Could you check a few things on this model? Use its own coordinates, in mm. A direction names the side the tool comes from. Round coordinates to 2 decimals unless told otherwise and drop trailing zeros. Loops run counter-clockwise (first coordinate to the right, second up) from the corner with the lowest first, then second, coordinate; pieces in that order, holes last. Notation, with made-up numbers: M 55,66.25 L 113,66.25 A15 ccw 113,78.25 Z; hole C -0.75,-12 d9. An arc over 180 degrees is marked long. Answer in a Markdown table with one row per item.
Autodesk Inventor part; units mm, degrees
ref_plane "YZ Plane" through (0, 0, 0) normal (1, 0, 0) x (0, 1, 0)
ref_plane "XZ Plane" through (0, 0, 0) normal (0, 1, 0) x (-1, 0, 0)
ref_plane "XY Plane" through (0, 0, 0) normal (0, 0, 1) x (1, 0, 0)
sketch "DShaft" plane through (0, 0, 5) normal (0, 0, 1) x (1, 0, 0)
  circle A0 centre (0, 0) radius 4
  line L0 (-1.3919, 3.75) -> (1.3919, 3.75)
  dimension "d174" = 3.75
sketch "Sketch17" plane through (0, 0, 5) normal (0, 0, 1) x (1, 0, 0)
  arc A0 (55.3611, 0.3584) -> (42.3326, -1.2004) centre (50.1387, -11.2181) ccw
  arc A1 (55.3611, 0.3584) -> (35.2473, 5.0627) centre (33.3341, -48.4687) ccw
  arc A2 (25.4, -0.0141) -> (0, -25.4) centre (0, 0) ccw
  arc A3 (21.8139, 13.0121) -> (35.2473, 5.0627) centre (35.8302, 21.3728) ccw
  arc A4 (85.2601, -13.2441) -> (55.3611, 0.3584) centre (-2070.8473, -4712.7994) ccw
  arc A5 (25.4, -0.0141) -> (42.3326, -1.2004) centre (34.5266, 8.8174) ccw
sketch "Base" plane through (0, 0, 0) normal (0, 0, 1) x (1, 0, 0)
  circle A0 centre (0, 0) radius 25.4
  arc A1 (296.4611, -175.8738) -> (140.4514, -91.7589) centre (131.6761, -294.7694) ccw
  arc A2 (110.2711, -36.5273) -> (55.3611, 0.3584) centre (-26.1088, -180.2356) ccw
  arc A3 (110.2711, -36.5273) -> (151.7939, -57.2356) centre (164.9104, 21.0482) ccw
  arc A4 (244.1, -98.1325) -> (151.7939, -57.2356) centre (118.2154, -257.642) ccw
  arc A5 (244.1, -98.1325) -> (322.9398, -136.302) centre (369.9847, 61.3771) ccw
  arc A6 (339.7063, -172.5127) -> (322.9398, -136.302) centre (317.0592, -161.0119) ccw
  arc A7 (296.4611, -175.8738) -> (339.7063, -172.5127) centre (317.0592, -161.0119) ccw
  line L0 (128.6011, -96.3262) -> (140.4514, -91.7589)
  line L1 (0, 0) -> (317.0592, -161.0119) construction
  circle A8 centre (317.0592, -161.0119) radius 25.4 construction
  arc A9 (0, -25.4) -> (128.6011, -96.3262) centre (153.166, 100.265) ccw
  line L2 (0, 0) -> (0, -25.4) construction
  arc A10 (55.3611, 0.3584) -> (42.3326, -1.2004) centre (50.1387, -11.2181) ccw
  arc A11 (25.4, -0.0141) -> (42.3326, -1.2004) centre (34.5266, 8.8174) ccw
  line L3 (110.2711, -36.5273) -> (102.4101, -52.0068) construction
  line L4 (50.1387, -11.2181) -> (44.3883, -22.5417) construction
  line L5 (140.4514, -91.7589) -> (148.7008, -75.5146) construction
  line L6 (244.1, -98.1325) -> (233.6726, -118.6658) construction
  line L7 (339.7063, -172.5127) -> (317.0592, -161.0119) construction
  dimension "d101" = 50.8
  dimension "d98" = 355.6
  dimension "d99" = 203.2
  dimension "d100" = 79.375
  dimension "d102" = 198.12
  dimension "d103" = 50.8
  dimension "d104" = 12.7
  dimension "d105" = 203.2
  dimension "d106" = 48
  dimension "d107" = 12.7
  dimension "d108" = 12.7
  dimension "d109" = 23.495
  dimension "d111" = 158.75
  dimension "d112" = 222.25
  dimension "d113" = 49.784
  dimension "d114" = 65.0748
  dimension "d115" = 51.9176
  dimension "d116" = 95.3008
  dimension "d117" = 93.5228
extrude "Plate1" add sketch "Base" along normal blind 5
sketch "MountHoles" plane through (0, 0, 5) normal (0, 0, 1) x (1, 0, 0)
  arc A0 (296.4611, -175.8738) -> (322.9398, -136.302) centre (317.0592, -161.0119) ccw
  circle A1 centre (317.0592, -161.0119) radius 3.175
  circle A2 centre (0, 0) radius 3.175
  circle A3 centre (0, 0) radius 15.875 construction
  circle A4 centre (0, 15.875) radius 3.175
  line L0 (0, 15.875) -> (0, 0) construction
  circle A5 centre (-13.7482, 7.9375) radius 3.175
  circle A6 centre (-13.7482, -7.9375) radius 3.175
  circle A7 centre (0, -15.875) radius 3.175
  circle A8 centre (13.7482, -7.9375) radius 3.175
  circle A9 centre (13.7482, 7.9375) radius 3.175
  point P0 (278.6053, -195.7416)
  point P1 (14.9365, 6.9557)
  dimension "d40" = 31.75
  dimension "d38" = 6.35
  dimension "d39" = 6.35
  dimension "d43" = 360
hole "MountHolesFeature" at (0, 0, 5) direction (0, 0, -1) diameter 8 end through all
fillet "SmallFilletsFeature" radius 8 2 edges at (140.4514, -91.7589, 2.5) (128.6011, -96.3262, 2.5)
sketch "WheelMountHole" plane through (0, 0, 5) normal (0, 0, 1) x (1, 0, 0)
  arc A0 (296.4611, -175.8738) -> (322.9398, -136.302) centre (317.0592, -161.0119) ccw
  circle A1 centre (317.0592, -161.0119) radius 6.35
  point P0 (0, 0)
  point P1 (278.6053, -195.7416)
  dimension "d83" = 12.7
hole "WheelMountHoleFeature" at (317.0592, -161.0119, 5) direction (0, 0, -1) diameter 24.5 end through all
sketch "PistonMountHole" plane through (0, 0, 0) normal (0, 0, -1) x (-1, 0, 0)
  circle A0 centre (-195.6083, -86.6143) radius 3
  arc A1 (-151.7939, -57.2356) -> (-244.1, -98.1325) centre (-118.2154, -257.642) ccw
  line L0 (-206.4619, -74.6043) -> (-184.7548, -98.6243) construction
  arc A2 (-142.169, -91.8405) -> (-296.4611, -175.8738) centre (-131.6761, -294.7694) ccw
  point P0 (0, 0)
  dimension "d120" = 6
  dimension "d122" = 203.2
extrude "PistonMountHoleFeature" cut sketch "PistonMountHole" against normal blind 5
sketch "MotorExtend" plane through (0, 0, 5) normal (0, 0, 1) x (1, 0, 0)
  circle A0 centre (70.2482, -45.9648) radius 36
  arc A1 (0, -25.4) -> (126.5447, -96.0583) centre (153.166, 100.265) ccw construction
  arc A2 (110.2711, -36.5273) -> (151.7939, -57.2356) centre (164.9104, 21.0482) ccw construction
  circle A3 centre (0, 0) radius 4
  line L0 (0, 0) -> (140.4963, -91.9296) construction
  arc A4 (142.169, -91.8405) -> (138.8789, -92.365) centre (141.7559, -99.8298) ccw
  arc A5 (0, -25.4) -> (46.966, -73.4228) centre (280.2614, 201.7164) ccw
  arc A6 (126.5447, -96.0583) -> (130.4966, -95.5956) centre (127.6196, -88.1308) ccw
  arc A7 (58.6335, -80.0397) -> (126.5447, -96.0583) centre (175.0163, 261.4034) ccw
  arc A8 (55.3611, 0.3584) -> (42.3326, -1.2004) centre (50.1387, -11.2181) ccw
  arc A9 (85.2601, -13.2441) -> (55.3611, 0.3584) centre (-2070.8473, -4712.7994) ccw
  arc A10 (110.2711, -36.5273) -> (55.3611, 0.3584) centre (-26.1088, -180.2356) ccw
  arc A11 (110.2711, -36.5273) -> (94.2542, -19.1374) centre (12.4591, -110.5454) ccw
  line L1 (0, -25.4) -> (55.3611, 0.3584)
  line L2 (110.2711, -36.5273) -> (126.5447, -96.0583)
  point P0 (70.2482, -45.9648)
  dimension "d128" = 72
sheet face with bend "MotorExtendFeature" sketch "MotorExtend" thickness 5 toward (0, 0, -1) bend radius 5 contours A0 A10 | A11 A10 A0 | A0 A10 A9 | A10 L2 A7 A0 | A0 A10 | A0 A5 L1 A10
bend "Bend1"
sketch "MotorCut" plane through (0, 0, 5) normal (0, 0, 1) x (1, 0, 0)
  circle A0 centre (70.2482, -45.9648) radius 36
  circle A1 centre (70.2482, -45.9648) radius 15
  point P0 (0, 0)
  dimension "d134" = 30
extrude "MotorCutFeature" cut sketch "MotorCut" against normal blind 5 contours A1
sketch "MotorMountHoles" plane through (0, 0, 5) normal (0, 0, 1) x (1, 0, 0)
  circle A0 centre (56.943, -61.9327) radius 3.5
  circle A1 centre (63.0721, -26.4582) radius 3.5
  circle A2 centre (90.7293, -49.5034) radius 3.5
  point P0 (0, 0)
extrude "MotorMountHolesFeature" cut sketch "MotorMountHoles" against normal blind 5
sketch "HubCoverExtend" plane through (0, 0, 5) normal (0, 0, 1) x (1, 0, 0)
  circle A0 centre (317.0592, -161.0119) radius 12.25
  circle A1 centre (317.0592, -161.0119) radius 50.8
  arc A2 (244.1, -98.1325) -> (322.9398, -136.302) centre (369.9847, 61.3771) ccw
  arc A3 (296.4611, -175.8738) -> (142.169, -91.8405) centre (131.6761, -294.7694) ccw
  arc A4 (244.1, -98.1325) -> (305.2545, -111.6025) centre (288.573, -41.7804) ccw
  arc A5 (266.9914, -169.606) -> (228.8665, -116.3198) centre (192.9202, -182.3202) ccw
  point P0 (0, 0)
  point P1 (283.7795, -122.6308)
  point P2 (268.8853, -144.8899)
  dimension "d139" = 101.6
sheet face with bend "HubCoverExtendFeature" sketch "HubCoverExtend" thickness 5 toward (0, 0, -1) bend radius 5
bend "Bend2"
sketch "HubPressFitHole" plane through (0, 0, 5) normal (0, 0, 1) x (1, 0, 0)
  circle A0 centre (317.0592, -161.0119) radius 12.25
  circle A1 centre (317.0592, -161.0119) radius 35.9873
  point P0 (0, 0)
  dimension "d145" = 71.9746
extrude "HubPressFitHoleFeature" cut sketch "HubPressFitHole" against normal blind 5 contours A0 | A1
sketch "ShinThicken" plane through (0, 0, 5) normal (0, 0, 1) x (1, 0, 0)
  arc A0 (266.9914, -169.606) -> (228.8665, -116.3198) centre (192.9202, -182.3202) ccw
  arc A1 (228.8665, -116.3198) -> (142.169, -91.8405) centre (131.6761, -294.7694) ccw
  arc A2 (266.9914, -169.606) -> (142.169, -91.8405) centre (133.4629, -244.8745) ccw
  point P0 (0, 0)
sheet face with bend "ShinThickenFeature" sketch "ShinThicken" thickness 5 toward (0, 0, -1) bend radius 5
bend "Bend3"
fillet "BlendFilletFeature" radius 32 1 edges at (266.9914, -169.606, 2.5)
sheet face with bend "DShaftFeature" sketch "DShaft" thickness 5 toward (0, 0, -1) bend radius 5 picked at (-0.1576, 3.824) contours L0 A0
bend "Bend6"
equation "\"d66\" = Thickness"
equation "\"d89\" = Thickness"
equation "\"d37\" = Thickness"
equation "\"BendRadius\" = Thickness"
equation "\"BendReliefWidth\" = Thickness"
equation "\"BendReliefDepth\" = 0.5 * Thickness"
equation "\"TransitionRadius\" = BendRadius"
equation "\"JacobiRadiusSize\" = BendRadius"
equation "\"GapSize\" = Thickness"
properties part number "LowerLeg"
1) I need wall thicknesses on line 1 (Y direction, x = 0, z = 2.4); line 2 (X direction, y = -133, z = 3.85); line 3 (X direction, y = -158, z = 4.05). Which ranges of each line are inside material? Lowest first, please.
Computed:
| item | result |
|---|---|
| line 1 | y = -25.4 to -4, 3.75 to 25.4 |
| line 2 | x = 238.25 to 294.47, 339.65 to 359.44 |
| line 3 | x = 259.75 to 281.2, 352.92 to 367.77 |
2) I want a section at C-C, the plane x = 119. Please give me the cut outline in (y, z).
Computed:
| item | result |
|---|---|
| outline | M -94.95,0 L -43.7,0 L -43.7,5 L -94.95,5 Z |
3) I want a section at B-B, the plane z = 3.85. State how many separate pieces and enclosed holes the cut face has, plus the area to 3 significant figures.
Computed:
| item | result |
|---|---|
| separate pieces | 1 |
| enclosed holes | 7 |
| area | 18,300 mm² |
4) Will these pins go through, and if not, where does the flat tip stop? P1, Ø18, axis at x = 70.25, y = -45.96, coming from the -Z side; P2, Ø1.5, axis at x = 273.5, z = 2.5, coming from the +Y side; P3, Ø1.5, axis at x = 210.5, z = 1, coming from the +Y side; P4, Ø3, axis at x = 0, z = 2, coming from the -Y side.
Computed:
| item | result |
|---|---|
| P1 | passes through |
| P2 | stops at y = -111.8 |
| P3 | stops at y = -76.23 |
| P4 | stops at y = -27.24 |
5) Which directions (+Z, -Z, +X, -X, +Y, -Y) give clear straight access to the entire face, cutting with the end or side of a thin tool? Please do faces 1 (the face through (67, -60.61, 2.54)), 2 (the face through (212.949, -113.813, 2.535)).
Computed:
| item | result |
|---|---|
| face 1 | +Z, -Z |
| face 2 | +Z, -Z, -Y |
6) I want a section at A-A, the plane y = -181. Please give me the cut outline in (x, z), plus the area to 3 significant figures.
Computed:
| item | result |
|---|---|
| outline | M 270.36,0 L 287.13,0 L 287.13,5 L 270.36,5 Z; M 346.99,0 L 363.76,0 L 363.76,5 L 346.99,5 Z |
| area | 168 mm² |
7) If we mould it in two halves opening along X, with no side actions, what happens to faces 3 (the face through (58.558, -65.038, 2.535)), 4 (the face through (156, -84, 5)), 5 (the face through (0, -4, 2)), 6 (the face through (22.034, -50.17, 2.535))? For each: released by +X, released by -X, zero draft, split by the parting line, or undercut.
Computed:
| item | result |
|---|---|
| face 3 | undercut |
| face 4 | zero draft |
| face 5 | undercut |
| face 6 | released by -X |
8) I want a section at D-D, the plane y = -120.5. Please give me the cut outline in (x, z).
Computed:
| item | result |
|---|---|
| outline | M 223.05,0 L 347.71,0 L 347.71,5 L 223.05,5 Z |
